```python
from build123d import *

# Parameters (mm, degrees)
F1_DEPTH    = 6.35
F2_R        = 5.08
F3_T1_DEPTH = 19.2442405969
F3_T4_ANGLE = 180
F3_T6_ANGLE = 180


# Not quite as in the source:
# - a fillet or chamfer that OpenCascade refuses, or shapes differently, is made with other operations: its cross-section is extruded or revolved along the edge and cut away or added


with BuildPart() as f1:
    # F0 (on Top) → F1 (new body)
    with BuildSketch(Plane.XY):
        with BuildLine():
            Line((20.5361241051, 0), (20.5361241051, 19.2442405969))
            ThreePointArc((20.5361241051, 19.2442405969), (0, 39.780364702), (-20.5361241051, 19.2442405969))
            Line((-20.5361241051, 19.2442405969), (-20.5361241051, 0))
            ThreePointArc((-20.5361241051, 0), (0, -20.5361241051), (20.5361241051, 0))
        make_face()
        with BuildLine():
            ThreePointArc((14.1861241051, 0), (0, -14.1861241051), (-14.1861241051, 0))
            Line((-14.1861241051, 0), (-14.1861241051, 19.2442405969))
            ThreePointArc((-14.1861241051, 19.2442405969), (0, 33.430364702), (14.1861241051, 19.2442405969))
            Line((14.1861241051, 19.2442405969), (14.1861241051, 0))
        make_face(mode=Mode.SUBTRACT)
    extrude(amount=F1_DEPTH)

    # F2
    f2_edges = [f1.edges().sort_by_distance(p)[0] for p in [
        (0, 39.780365, 6.35),
    ]]
    fillet(f2_edges, radius=F2_R)

    # F3: fillet of radius 5.08 on 1 edges, made by hand

    # F3_s2 → F3_t1 (cut)
    with BuildSketch(Plane.XZ.offset(-19.2442405969)):
        with BuildLine():
            ThreePointArc((20.5361241051, 1.27), (18.9720711643, 0.3280951188), (17.1760199401, 0))
            Line((17.1760199401, 0), (20.5361241051, 0))
            Line((20.5361241051, 0), (20.5361241051, 1.27))
        make_face()
        with BuildLine():
            ThreePointArc((-17.1760199401, 0), (-18.9720711643, 0.3280951188), (-20.5361241051, 1.27))
            Line((-20.5361241051, 1.27), (-20.5361241051, 0))
            Line((-20.5361241051, 0), (-17.1760199401, 0))
        make_face()
    extrude(amount=F3_T1_DEPTH, mode=Mode.SUBTRACT)

    # F3_s3 → F3_t4 (revolve, cut)
    with BuildSketch(Plane.XZ.offset(-19.2442405969)):
        with BuildLine():
            ThreePointArc((17.1760199401, 0), (18.9720711643, 0.3280951188), (20.5361241051, 1.27))
            Line((20.5361241051, 1.27), (20.5361241051, 0))
            Line((20.5361241051, 0), (17.1760199401, 0))
        make_face()
    revolve(axis=Axis((0, 19.2442405969, 0), (0, 0, 1)), revolution_arc=F3_T4_ANGLE, mode=Mode.SUBTRACT)

    # F3_s5 → F3_t6 (revolve, cut)
    with BuildSketch(Plane.XZ):
        with BuildLine():
            ThreePointArc((-20.5361241051, 1.27), (-18.9720711643, 0.3280951188), (-17.1760199401, 0))
            Line((-17.1760199401, 0), (-20.5361241051, 0))
            Line((-20.5361241051, 0), (-20.5361241051, 1.27))
        make_face()
    revolve(axis=Axis((0, 0, 0), (0, 0, 1)), revolution_arc=F3_T6_ANGLE, mode=Mode.SUBTRACT)


solid = f1.part
```
Build history of the part. All positions in model axes, mm. A direction names the side the tool comes from. Round coordinates to 2 decimals unless told otherwise and drop trailing zeros. Order: outer loops, then holes, each group sorted by start corner. A loop starts at its lowest first (then second) coordinate and runs counter-clockwise, first axis right, second up. Notation, with made-up numbers: (-32.5, 19.25) - (-7.5, 19.25) arc R34 cw to (-7.5, 56.25) - close; hole circle Ø3 at (-25, 30). An arc over 180 degrees is marked (long way). Use a Markdown table: item, result.
1) Tool access for faces 1 (the face through (-15, 10, 6.35)), 2 (the face through (0.312, -14.183, 3.131)): list every direction of +Z, -Z, +X, -X, +Y, -Y with a clear straight run to the whole face (end or side of a thin tool).
Recorded:
| item | result |
|---|---|
| face 1 | +Z, +X, -X, +Y, -Y |
| face 2 | +Z, -Z |
2) Saw through at B-B on z = 2.75. Write the cut outline in (x, y).
Recorded:
| item | result |
|---|---|
| outline | (-20.32, 0) arc R20.32 ccw to (20.32, 0) - (20.32, 19.24) arc R20.32 ccw to (-20.32, 19.24) - close; hole (-14.19, 0) arc R14.19 ccw to (14.19, 0) - (14.19, 19.24) arc R14.19 ccw to (-14.19, 19.24) - close |
3) Pull direction X, two halves, no side cores. Call faces 3 (the face through (-14.186, 9, 3)), 4 (the face through (-19.09, 9.49, 4.82)), 5 (the face through (19, 9.76, 0.34)), 6 (the face through (-0.312, 33.427, 3.131)): pulls with the +X half, pulls with the -X half, needs draft (parallel to the pull), parting line crosses it, or undercut.
Recorded:
| item | result |
|---|---|
| face 3 | undercut |
| face 4 | pulls with the -X half |
| face 5 | pulls with the +X half |
| face 6 | undercut |
4) Flat gauge pins, fed straight in: pin 1 Ø2 at (y, z) = (-13.5, 4.5) entering from -X; pin 2 Ø8 at (x, y) = (-8.5, 1) entering from +Z; pin 3 Ø1 at (x, z) = (11, 1) entering from +Y; pin 4 Ø1.5 at (y, z) = (19.5, 4) entering from +X. Where does each tip first touch, or does it go through?
Recorded:
| item | result |
|---|---|
| pin 1 | stops at x = -15.2 |
| pin 2 | passes through |
| pin 3 | stops at y = 36.85 |
| pin 4 | stops at x = 20.13 |
5) Saw through at A-A on x = 0. Write the cut outline in (y, z).
Recorded:
| item | result |
|---|---|
| outline | (-20.54, 1.27) arc R5.08 ccw to (-17.18, 0) - (-14.19, 0) - (-14.19, 6.35) - (-15.46, 6.35) arc R5.08 ccw to start; (33.43, 0) - (36.42, 0) arc R5.08 ccw to (39.78, 1.27) arc R5.08 ccw to (34.7, 6.35) - (33.43, 6.35) - close |
6) Wall check: L1, parallel to Y at x = -4, z = 4.25; L2, parallel to X at y = -5.5, z = 5.5; L3, parallel to Y at x = 13, z = 3.25. Give the ranges that are in metal, low to high.
Recorded:
| item | result |
|---|---|
| L1 | y = -19.16 to -13.61, 32.85 to 38.4 |
| L2 | x = -17.42 to -13.08, 13.08 to 17.42 |
| L3 | y = -15.38 to -5.68, 24.92 to 34.62 |
